Check sheet for the modelled part. Datum: model origin and axes. Units: mm. A direction names the side the tool comes from. Round coordinates to 2 decimals unless told otherwise and drop trailing zeros. Order: outer loops, then holes, each group sorted by start corner. A loop starts at its lowest first (then second) coordinate and runs counter-clockwise, first axis right, second up.
(1) Sectioned sample at B-B, the plane y = 42.5. Enter the section's corners in (x, z).
(2) Mould release check, pull along Z, two halves, no side actions. Record for faces 6 (the flat face through (5, 49.53, 5)), 7 (the cylindrical face through (-0.33, 15.85, 2.52)), 8 (the flat face through (9.783, -6.261, 5.271)): released by +Z, released by -Z, zero draft, split by the parting line, or undercut.
(3) Thickness scan on probe 1 along Z at (x, y) = (0, 12.5) (3 decimals); probe 2 along Z at (x, y) = (0, 33). Record the ranges inside material, lowest first.
(4) Sectioned sample at A-A, the plane x = 0. Enter the section's corners in (y, z) (3 decimals), and give its area (3 significant figures).
(5) Sectioned sample at C-C, the plane y = 11. Enter the section's corners in (x, z) (3 decimals), and give its area (3 significant figures).
(6) Depth check by flat-ended pin: pin 1 (2 mm diameter, centred on x = 6.5, y = 7, fed in from -Z); pin 2 (1 mm diameter, centred on y = 20.5, z = 10, fed in from +X); pin 3 (10 mm diameter, centred on x = -12, y = 39, fed in from -Z). Enter the tip coordinate at first touch or a pass-through.
(7) Tool access check on faces 1 (the cylindrical face through (-13.02, 36.41, -4.1)), 2 (the flat face through (-9.456, -6.261, 5.837)), 3 (the flat face through (9.456, -6.261, -5.837)), 4 (the flat face through (-9.783, -6.261, -5.271)), 5 (the flat face through (-11, 0, 5)). Record the directions out of +Z, -Z, +X, -X, +Y, -Y that give a thin tool (end or side, any length) a straight path to the whole face; none if there is none.
```python
from build123d import *

# Parameters (mm, degrees)
BOSS_EXTRUDE2_DEPTH = 12.7
CHAMFER2_SIZE       = 2.413
SKETCH13_R          = 2.54
CUT_EXTRUDE1_DEPTH  = 63.23


with BuildPart() as part:
    # Sketch1 → Revolve1 (revolve)
    with BuildSketch(Plane.XY):
        Polygon((-15.875, 25.4), (-13.64869, 25.4), (-13.64869, 49.53), (-6.858, 49.53), (0, 42.672), (0, 0), (-15.875, 0), align=None)
    revolve(axis=Axis((0, 110.151211274, 0), (0, -1, 0)))

    # Sketch12 → Boss-Extrude2 (add)
    with BuildSketch(Plane.XZ):
        Polygon((-12.828682674, 0.274060562), (-6.651684746, -10.972934812), (6.176997928, -11.246995373), (12.828682674, -0.274060562), (6.651684746, 10.972934812), (-6.176997928, 11.246995373), align=None)
    extrude(amount=BOSS_EXTRUDE2_DEPTH)

    # Chamfer2
    chamfer2_edges = [part.edges().sort_by_distance(p)[0] for p in [
        (13.64869, 49.53, 0),
    ]]
    chamfer(chamfer2_edges, length=CHAMFER2_SIZE)

    # Sketch13 → Cut-Extrude1 (cut, through all)
    with BuildSketch(Plane.XZ.offset(12.7)):
        Circle(SKETCH13_R)
    extrude(amount=-CUT_EXTRUDE1_DEPTH, mode=Mode.SUBTRACT)


solid = part.part
```
Derived:
1. outline: circle Ø27.3 at (0, 0); hole circle Ø5.08 at (0, 0)
2. face 6: zero draft
2. face 7: undercut
2. face 8: released by +Z
3. probe 1: z = -15.875 to -2.54, 2.54 to 15.875
3. probe 2: z = -13.65 to -2.54, 2.54 to 13.65
4. outline: (-12.7, -11.115) - (0, -11.115) - (0, -15.875) - (25.4, -15.875) - (25.4, -13.649) - (47.117, -13.649) - (49.53, -11.236) - (49.53, -6.858) - (45.212, -2.54) - (-12.7, -2.54) - close; (-12.7, 2.54) - (45.212, 2.54) - (49.53, 6.858) - (49.53, 11.236) - (47.117, 13.649) - (25.4, 13.649) - (25.4, 15.875) - (0, 15.875) - (0, 11.115) - (-12.7, 11.115) - close
4. area: 1,410 mm2
5. outline: circle Ø31.75 at (0, 0); hole circle Ø5.08 at (0, 0)
5. area: 771 mm2
6. pin 1: stops at z = -14.89
6. pin 2: stops at x = 12.72
6. pin 3: stops at z = -11.72
7. face 1: +Y
7. face 2: +Z, -X, -Y
7. face 3: -Z, +X, -Y
7. face 4: -Z, -X, -Y
7. face 5: -Y
